from build123d import *

# Parameters (mm, degrees)
F0_R     = 5
F0_R_2   = 6
F0_R_3   = 7
F1_DEPTH = 25


with BuildPart() as f1:
    # F0 (on Front) → F1 (new body, symmetric)
    with BuildSketch(Plane.XZ):
        with BuildLine():
            ThreePointArc((-5.553130951, -8.3164136887), (-4.7153308734, 8.8184836993), (10, 0))
            ThreePointArc((10, 0), (8.5065080835, -5.2573111212), (4.472135955, -8.94427191))
            Line((4.472135955, -8.94427191), (44.472135955, 11.05572809))
            ThreePointArc((44.472135955, 11.05572809), (31.05572809, 15.527864045), (35.527864045, 28.94427191))
            Line((35.527864045, 28.94427191), (16.6647048429, 19.512692309))
            ThreePointArc((16.6647048429, 19.512692309), (-3.1646914629, 17.0389630488), (-20.1486854537, 27.5683620073))
            Line((-20.1486854537, 27.5683620073), (-37.911559077, 49.7015254497))
            ThreePointArc((-37.911559077, 49.7015254497), (-35.3777424057, 45.1419434893), (-34.5, 40))
            ThreePointArc((-34.5, 40), (-42.6912371463, 26.3313502661), (-58.607352974, 27.1095587825))
            Line((-58.607352974, 27.1095587825), (-5.553130951, -8.3164136887))
        make_face()
        with BuildLine():
            ThreePointArc((-37.911559077, 49.7015254497), (-61.4292927515, 50.4700175358), (-58.607352974, 27.1095587825))
            ThreePointArc((-58.607352974, 27.1095587825), (-42.6912371463, 26.3313502661), (-34.5, 40))
            ThreePointArc((-34.5, 40), (-35.3777424057, 45.1419434893), (-37.911559077, 49.7015254497))
        make_face()
        with Locations((-50, 40)):
            Circle(F0_R, mode=Mode.SUBTRACT)
        with BuildLine():
            ThreePointArc((4.472135955, -8.94427191), (8.5065080835, -5.2573111212), (10, 0))
            ThreePointArc((10, 0), (-4.7153308734, 8.8184836993), (-5.553130951, -8.3164136887))
            ThreePointArc((-5.553130951, -8.3164136887), (-0.6250512234, -9.9804464313), (4.472135955, -8.94427191))
        make_face()
        Circle(F0_R_2, mode=Mode.SUBTRACT)
        with BuildLine():
            ThreePointArc((35.527864045, 28.94427191), (31.05572809, 15.527864045), (44.472135955, 11.05572809))
            ThreePointArc((44.472135955, 11.05572809), (48.5065080835, 14.7426888788), (50, 20))
            ThreePointArc((50, 20), (45.2573111212, 28.5065080835), (35.527864045, 28.94427191))
        make_face()
        with Locations((40, 20)):
            Circle(F0_R_3, mode=Mode.SUBTRACT)
    extrude(amount=F1_DEPTH, both=True)


solid = f1.part
For this review, take the finished solid that the model builds, in its own axes (mm). A direction names the side the tool comes from. Round coordinates to 2 decimals unless told otherwise and drop trailing zeros. Loops run counter-clockwise (first coordinate to the right, second up) from the corner with the lowest first, then second, coordinate; pieces in that order, holes last. Notation, with made-up numbers: (19, 49.25) - (69, 49.25) arc R20 cw to (69, 53.25) - close; hole circle Ø3 at (34, 24.25). An arc over 180 degrees is marked (long way). Use one line per item in the form item = value.
1) We need section D-D on z = 40. Write out the cut boundary in (x, y), then the cut area to 3 significant figures.
Solutions:
outline = (-65.5, -25) - (-55, -25) - (-55, 25) - (-65.5, 25) - close; (-45, -25) - (-30.13, -25) - (-30.13, 25) - (-45, 25) - close
area = 1,270 mm2
2) Wall thickness on probe 1 along Z at (x, y) = (-48.5, 3.5); probe 2 along X at (y, z) = (-3.5, 4); probe 3 along Z at (x, y) = (0, -7): over which ranges is each line inside the solid? List them lowest first.
Solutions:
probe_1 = 20.36 to 35.23, 44.77 to 55.43
probe_2 = -24 to -4.47, 4.47 to 30.36
probe_3 = -10 to -6, 6 to 16.52
3) Tool access review of faces 1 (the face through (-61.173, -0.35, 50.743)), 2 (the face through (26.228, -0.35, 24.295)): name each direction out of +Z, -Z, +X, -X, +Y, -Y from which nothing blocks a thin tool from reaching the whole face with its end or side.
Solutions:
face_1 = +Y, -Y
face_2 = +Z, +Y, -Y
4) We need section A-A on x = -51. Write out the cut boundary in (y, z).
Solutions:
outline = (-25, 22.03) - (25, 22.03) - (25, 35.1) - (-25, 35.1) - close; (-25, 44.9) - (25, 44.9) - (25, 55.47) - (-25, 55.47) - close
5) Clearance check with flat-ended pins moving along their axes: P1, Ø5, axis at y = 2.5, z = 47, coming from the -X side; P2, Ø1.5, axis at y = -1, z = -1, coming from the +X side; P3, Ø8, axis at x = -19.5, y = -15.5, coming from the +Z side. State where each tip first meets the part, or that it passes through.
Solutions:
P1 = -64.83
P2 = 21.86
P3 = 31.74
6) Mouldability with a two-part tool opening along Z and no side actions: class faces 3 (the face through (-17, -25, 20)), 4 (the face through (-32.452, -0.35, 9.645)), 5 (the face through (-6, 0, 0)) as pulls with the +Z half, pulls with the -Z half, needs draft (parallel to the pull), parting line crosses it, or undercut.
Solutions:
face_3 = needs draft
face_4 = pulls with the -Z half
face_5 = undercut
7) We need section C-C on z = 18. Write out the cut boundary in (x, y), then the cut area to 3 significant figures.
Solutions:
outline = (-44.96, -25) - (-6.58, -25) - (-6.58, 25) - (-44.96, 25) - close; (13.07, -25) - (33.29, -25) - (33.29, 25) - (13.07, 25) - close; (46.71, -25) - (49.8, -25) - (49.8, 25) - (46.71, 25) - close
area = 3,080 mm2
8) We need section B-B on y = -5. Write out the cut boundary in (x, z), then the cut area to 3 significant figures.
Solutions:
outline = (-58.61, 27.11) - (-5.55, -8.32) arc R10 ccw to (4.47, -8.94) - (44.47, 11.06) arc R10 ccw to (35.53, 28.94) - (16.66, 19.51) arc R30 cw to (-20.15, 27.57) - (-37.91, 49.7) arc R15.5 ccw (long way) to start; hole circle Ø10 at (-50, 40); hole circle Ø12 at (0, 0); hole circle Ø14 at (40, 20)
area = 2,630 mm2
